Model file for the job. Use its own axes, mm. Round coordinates to 2 decimals unless told otherwise and drop trailing zeros. Write each loop counter-clockwise with the first axis right and the second up, starting at its lowest first coordinate (ties: lowest second). Pieces come first, ordered by that corner, then holes. Notation, with made-up numbers: (29.25, -18.75) - (73.25, -18.75) arc R18 ccw to (73.25, 8.25) - close; hole circle Ø6 at (31.25, -26.75). An arc over 180 degrees is marked (long way). One line per item, written item: value.
Autodesk Inventor part; units mm, degrees
ref_plane "YZ Plane" through (0, 0, 0) normal (1, 0, 0) x (0, 1, 0)
ref_plane "XZ Plane" through (0, 0, 0) normal (0, 1, 0) x (-1, 0, 0)
ref_plane "XY Plane" through (0, 0, 0) normal (0, 0, 1) x (1, 0, 0)
sketch "Sketch1" plane through (0, 0, 0) normal (1, 0, 0) x (0, 1, 0)
  circle A0 centre (0, 0) radius 2.5527
  line L0 (7.3323, 0) -> (3.6662, -6.35)
  line L1 (3.6662, -6.35) -> (-3.6662, -6.35)
  line L2 (-3.6662, -6.35) -> (-7.3323, 0)
  line L3 (-7.3323, 0) -> (-3.6662, 6.35)
  line L4 (-3.6662, 6.35) -> (3.6662, 6.35)
  line L5 (3.6662, 6.35) -> (7.3323, 0)
  point P0 (0, -6.35)
  dimension "d1" = 12.7
  dimension "d5" = 5.1054
extrude "Extrusion1" add sketch "Sketch1" along normal mid plane 28.5242
properties part number "1.123 hex shaft 0.25-20 0.5" material "Aluminum 6061"
1. Band-saw the part on C-C on z = -0.75. Write the cut outline in (x, y), plus the area to 3 significant figures.
Report:
outline: (-14.26, -6.9) - (14.26, -6.9) - (14.26, -2.44) - (-14.26, -2.44) - close; (-14.26, 2.44) - (14.26, 2.44) - (14.26, 6.9) - (-14.26, 6.9) - close
area: 254 mm²
2. Band-saw the part on A-A on x = -1.5. Write the cut outline in (y, z), plus the area to 3 significant figures.
Report:
outline: (-7.33, 0) - (-3.67, -6.35) - (3.67, -6.35) - (7.33, 0) - (3.67, 6.35) - (-3.67, 6.35) - close; hole circle Ø5.11 at (0, 0)
area: 119 mm²
3. Wall check: probe 1 along Z at (x, y) = (-3, 0); probe 2 along Z at (x, y) = (1.5, 1.75); probe 3 along Y at (x, z) = (-1.5, 3.5). Give the ranges that are in metal, low to high. Write a range as [from, to].
Report:
probe 1: [-6.35, -2.55], [2.55, 6.35]
probe 2: [-6.35, -1.86], [1.86, 6.35]
probe 3: [-5.31, 5.31]
4. Band-saw the part on B-B on y = 0. Write the cut outline in (x, z), plus the area to 3 significant figures.
Report:
outline: (-14.26, -6.35) - (14.26, -6.35) - (14.26, -2.55) - (-14.26, -2.55) - close; (-14.26, 2.55) - (14.26, 2.55) - (14.26, 6.35) - (-14.26, 6.35) - close
area: 217 mm²
5. Drop flat-ended pins along their axis: pin 1 (3 mm diameter, centred on y = 0, z = 0, fed in from -X); pin 2 (6 mm diameter, centred on x = 3.5, z = 5, fed in from +Y). Give the stop position or say it passes through.
Report:
pin 1: through
pin 2: y = 6.18
6. Mould opens along Z. For faces 1 (the face through (-0.2, 2.435, -0.767)), 2 (the face through (-0.2, 5.474, 3.219)), 3 (the face through (-14.262, 3, 0)) say: released by +Z, released by -Z, zero draft, split by the parting line, or undercut.
Report:
face 1: undercut
face 2: released by +Z
face 3: zero draft
7. Band-saw the part on D-D on y = 6.5. Write the cut outline in (x, z), plus the area to 3 significant figures.
Report:
outline: (-14.26, -1.44) - (14.26, -1.44) - (14.26, 1.44) - (-14.26, 1.44) - close
area: 82.2 mm²
